Answer from the drawing. Dimensions are ordinates in mm from the lowest x, y and z of the part. Coordinates: 2 decimals unless noted, no trailing zeros. Loops run counter-clockwise (first coordinate to the right, second up) from the corner with the lowest first, then second, coordinate; pieces in that order, holes last. Notation, with made-up numbers: (16.5, 6.25) -> (25.5, 6.25) arc R5 ccw to (25.5, 12.25) -> close; hole circle Ø8 at (18, 76). An arc over 180 degrees is marked (long way). Answer as CSV lines item,"result".
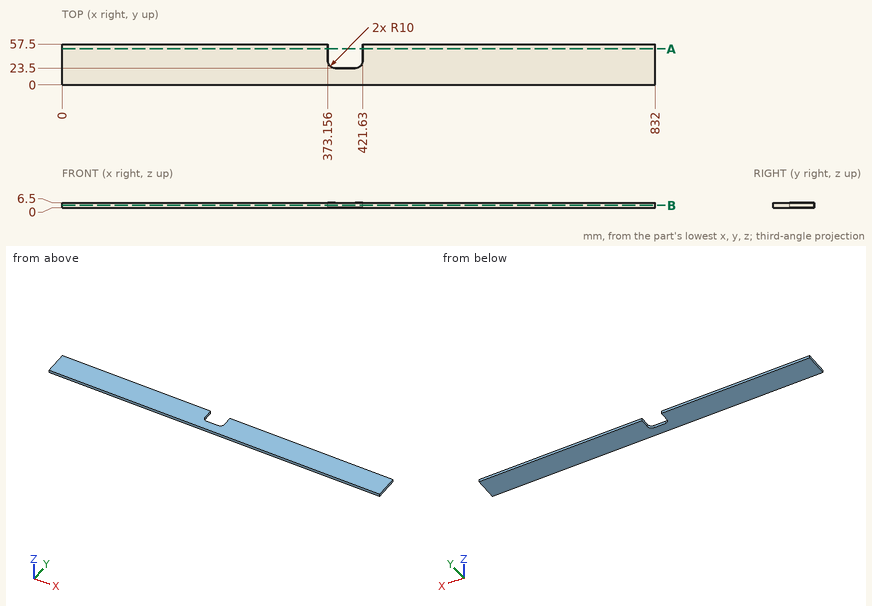
(1) A cutting plane is placed at A-A, the plane y = 50.5. Write down the section's boundary in (x, z), and give its area (3 significant figures).
Computed values:
outline,"(0, 0) -> (373.16, 0) -> (373.16, 6.5) -> (0, 6.5) -> close; (421.63, 0) -> (832, 0) -> (832, 6.5) -> (421.63, 6.5) -> close"
area,"5,090 mm2"
(2) A flat-ended cylindrical pin translates along its axis: pin 1 Ø3 at (x, z) = (391.5, 3) entering from +Y. Find the tip coordinate at first contact, or state that the pin passes through.
Computed values:
pin 1,"y = 23.5"
(3) Consider line 1 along X through (y, z) = (39.5, 4); line 2 along X through (y, z) = (28, 0.75). Determine where each line is inside the solid, lowest interval first.
Computed values:
line 1,"0 to 373.16, 421.63 to 832"
line 2,"0 to 374.8, 419.98 to 832"
(4) A cutting plane is placed at B-B, the plane z = 3. Write down the section's boundary in (x, y), and give its area (3 significant figures).
Computed values:
outline,"(0, 0) -> (832, 0) -> (832, 57.5) -> (421.63, 57.5) -> (421.63, 33.5) arc R10 cw to (411.63, 23.5) -> (383.16, 23.5) arc R10 cw to (373.16, 33.5) -> (373.16, 57.5) -> (0, 57.5) -> close"
area,"46,200 mm2"
